Source: three-view drawing plus pictorial views. Frame: mm from the lowest corner of the part. A direction names the side the tool comes from. Round coordinates to 2 decimals unless told otherwise and drop trailing zeros. Write each loop counter-clockwise with the first axis right and the second up, starting at its lowest first coordinate (ties: lowest second). Pieces come first, ordered by that corner, then holes. Notation, with made-up numbers: M -8.75,51 L -0.75,51 A10 cw -0.75,67 Z; hole C 85.25,50 d7. An arc over 180 degrees is marked long. Answer in a Markdown table with one row per item.
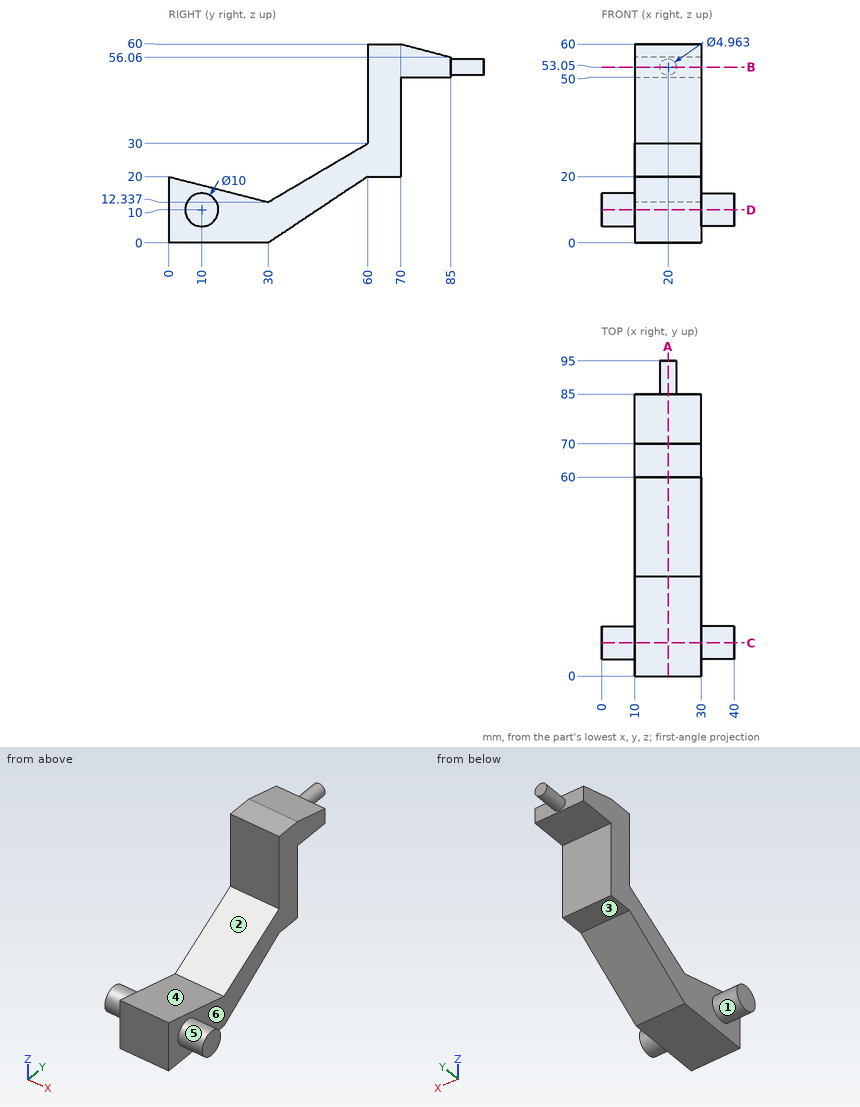
Q1. Section B-B (z = 53.05). Return loops of the section in (x, y).
Solutions:
| item | result |
|---|---|
| outline | M 10,60 L 30,60 L 30,85 L 22.48,85 L 22.48,95 L 17.52,95 L 17.52,85 L 10,85 Z |
Q2. Pull-direction query (Y, two-part tool) for the marked faces 4, 5 and 6; classes: pulls with the +Y half, pulls with the -Y half, needs draft (parallel to the pull), parting line crosses it, or undercut.
Solutions:
| item | result |
|---|---|
| face 4 | undercut |
| face 5 | parting line crosses it |
| face 6 | needs draft |
Q3. Contact query for flat-ended pins moving along their axis: pin 1 Ø1 at (x, z) = (11.5, 40) entering from -Y; pin 2 Ø3 at (x, y) = (10, 33.5) entering from +Z; pin 3 Ø16.5 at (x, y) = (23.5, 78) entering from -Z; pin 4 Ø1.5 at (x, y) = (8.5, 29) entering from +Z. Output: stop coordinate, or through.
Solutions:
| item | result |
|---|---|
| pin 1 | stops at y = 60 |
| pin 2 | stops at z = 15.28 |
| pin 3 | stops at z = 20 |
| pin 4 | passes through |
Q4. Access query for the marked faces 1, 2 and 3. Directions: +Z, -Z, +X, -X, +Y, -Y. A direction counts if a zero-diameter tool reaches every point of the face in a straight line with its end or side. Return the directions, or none.
Solutions:
| item | result |
|---|---|
| face 1 | -X |
| face 2 | +Z, +X, -X |
| face 3 | -Z, +X, -X, +Y |
Q5. Section D-D (z = 10). Return loops of the section in (x, y).
Solutions:
| item | result |
|---|---|
| outline | M 0,5 L 10,5 L 10,0 L 30,0 L 30,5 L 40,5 L 40,15 L 30,15 L 30,45 L 10,45 L 10,15 L 0,15 Z |
Q6. Section A-A (x = 20). Return loops of the section in (y, z), and give its area (3 significant figures).
Solutions:
| item | result |
|---|---|
| outline | M 0,0 L 30,0 L 60,20 L 70,20 L 70,50 L 85,50 L 85,50.57 L 95,50.57 L 95,55.53 L 85,55.53 L 85,56.06 L 70,60 L 60,60 L 60,30 L 30,12.34 L 0,20 Z |
| area | 1,390 mm2 |
Q7. Section C-C (y = 10). Return loops of the section in (x, z).
Solutions:
| item | result |
|---|---|
| outline | M 0,5 L 10,5 L 10,0 L 30,0 L 30,5 L 40,5 L 40,15 L 30,15 L 30,17.45 L 10,17.45 L 10,15 L 0,15 Z |
Q8. Material intervals for probe 1 along Z at (x, y) = (8, 10); probe 2 along X at (y, z) = (50.5, 15); probe 3 along Z at (x, y) = (18, 67), sorted ascending.
Solutions:
| item | result |
|---|---|
| probe 1 | z = 5 to 15 |
| probe 2 | x = 10 to 30 |
| probe 3 | z = 20 to 60 |
